```python
from build123d import *

# Parameters (mm, degrees)
F0_R     = 3.175
F1_DEPTH = 0.635
F3_DEPTH = 1.016


with BuildPart() as f1:
    # F0 (on Front) → F1 (new body)
    with BuildSketch(Plane.XZ):
        with BuildLine():
            Line((28.402705, 22.225), (3.002705, 22.225))
            ThreePointArc((3.002705, 22.225), (-19.222295, 0), (3.002705, -22.225))
            Line((3.002705, -22.225), (28.402705, -22.225))
            ThreePointArc((28.402705, -22.225), (50.627705, 0), (28.402705, 22.225))
        make_face()
        with Locations((42.094897, 0)):
            Circle(F0_R, mode=Mode.SUBTRACT)
    extrude(amount=F1_DEPTH)

    # F2 (on face) → F3 (join)
    with BuildSketch(Plane.XZ.offset(0.635)):
        Polygon((9.984385, 22.225), (3.002705, -22.225), (12.413018, -22.225), (12.413018, -5.801737), (19.159222, -5.801737), (19.159222, -22.225), (28.402705, -22.225), (21.421025, 22.225), align=None)
        Polygon((19.159222, 0), (12.413018, 0), (15.78612, 13.897184), align=None, mode=Mode.SUBTRACT)
    extrude(amount=F3_DEPTH)


solid = f1.part
```
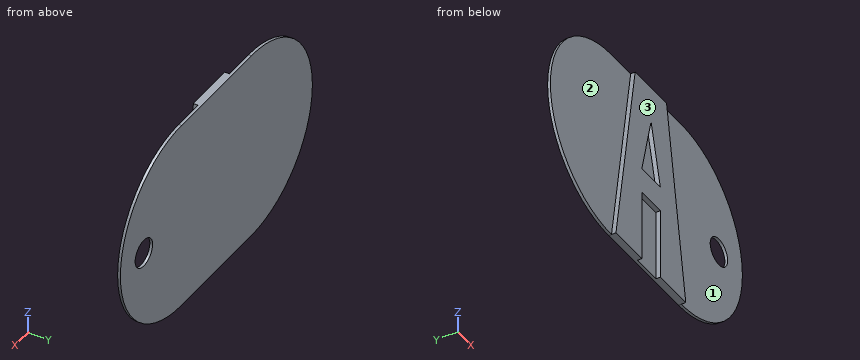
Could you check a few things on this model? Use its own coordinates, in mm. Face numbers are marked on the shaded views. A direction names the side the tool comes from. Round coordinates to 2 decimals unless told otherwise and drop trailing zeros. Loops run counter-clockwise (first coordinate to the right, second up) from the corner with the lowest first, then second, coordinate; pieces in that order, holes last. Notation, with made-up numbers: (45, 3) -> (68, 3) arc R22 cw to (68, 24) -> close; hole circle Ø7 at (25.5, -30). An arc over 180 degrees is marked (long way). One line per question, with ' | ' between items.
(1) If we section it at D-D on x = 17.5: List the corners of the cut face in (y, z) for me (3 decimals).
Model answer:
outline: (-1.651, -5.802) -> (-0.635, -5.802) -> (-0.635, -22.225) -> (0, -22.225) -> (0, 22.225) -> (-1.651, 22.225) -> (-1.651, 6.836) -> (-0.635, 6.836) -> (-0.635, 0) -> (-1.651, 0) -> close
(2) For the marked faces 1, 2 and 3, which set-ups out of +Z, -Z, +X, -X, +Y, -Y let a thin tool reach every point of the face, with its end or its side?
Model answer:
face 1: +Z, +X, -Y | face 2: +Z, -X, -Y | face 3: +Z, -Z, +X, -X, -Y
(3) If we section it at A-A on y = -0.95: List the corners of the cut face in (x, z) for me (3 decimals), and give its area (3 significant figures).
Model answer:
outline: (3.003, -22.225) -> (12.413, -22.225) -> (12.413, -5.802) -> (19.159, -5.802) -> (19.159, -22.225) -> (28.403, -22.225) -> (21.421, 22.225) -> (9.984, 22.225) -> close; hole (12.413, 0) -> (19.159, 0) -> (15.786, 13.897) -> close | area: 661 mm^2
(4) If I drill on probe 1 along Y at (x, z) = (2, -1) (3 decimals); probe 2 along X at (y, z) = (-0.95, -16.5); probe 3 along Z at (x, y) = (29, -0.4), over which ranges is the centre line in solid material (lowest first)?
Model answer:
probe 1: y = -0.635 to 0 | probe 2: x = 3.9 to 12.41, 19.16 to 27.5 | probe 3: z = -22.22 to 22.22
(5) If we section it at B-B on x = 43: List the corners of the cut face in (y, z) for me (3 decimals), and give its area (3 significant figures).
Model answer:
outline: (-0.635, -16.759) -> (0, -16.759) -> (0, -3.043) -> (-0.635, -3.043) -> close; (-0.635, 3.043) -> (0, 3.043) -> (0, 16.759) -> (-0.635, 16.759) -> close | area: 17.4 mm^2
(6) If we section it at C-C on z = 2.5: List the corners of the cut face in (x, y) for me (3 decimals), and give its area (3 significant figures).
Model answer:
outline: (-19.081, -0.635) -> (6.886, -0.635) -> (6.886, -1.651) -> (13.02, -1.651) -> (13.02, -0.635) -> (18.552, -0.635) -> (18.552, -1.651) -> (24.519, -1.651) -> (24.519, -0.635) -> (40.138, -0.635) -> (40.138, 0) -> (-19.081, 0) -> close; (44.052, -0.635) -> (50.487, -0.635) -> (50.487, 0) -> (44.052, 0) -> close | area: 54.0 mm^2
(7) For pin 1 Ø7.5 at (x, z) = (15, -15) entering from -Y; pin 2 Ø10 at (x, z) = (42.09, 0) entering from -Y (3 decimals), each with a flat end and sliding along its axis, tell me the tip position at first contact or that it passes through.
Model answer:
pin 1: stops at y = -1.65 | pin 2: stops at y = -0.635
